The model under review builds one solid part; all positions refer to its coordinate system, in mm. Face numbers are marked on the shaded views. Round coordinates to 2 decimals unless told otherwise and drop trailing zeros. Answer as a JSON object with one key per item and string values. Group by question number.
Item 1: The part is to be moulded in two halves that separate along Y. For the marked faces 1, 2, 3 and 4, say which applies: +Y half, -Y half, draft (parallel to the pull), parting line (faces both ways), or undercut.
Item 2: To check wall thickness, follow line 1 (Y direction, x = -14.5, z = 0); line 2 (Z direction, x = -11, y = -6); line 3 (Z direction, x = -10.5, y = 11.5). State the ranges of each line that lie inside material, in increasing order.
Item 3: Insertion check: P1, Ø3, axis at x = -10.5, y = 1, coming from the -Z side; P2, Ø3, axis at y = 13.5, z = 0, coming from the +X side; P3, Ø4, axis at x = -5, y = 6.5, coming from the -Z side; P4, Ø5.5, axis at y = 3, z = 1.5, coming from the +X side. Each pin has a flat end and moves straight along its axis. Give the tip position at first contact, or say it passes through.
Item 4: Consider section A-A (y = 1). State how many separate pieces and enclosed holes the cut face has, and give its area (3 significant figures).
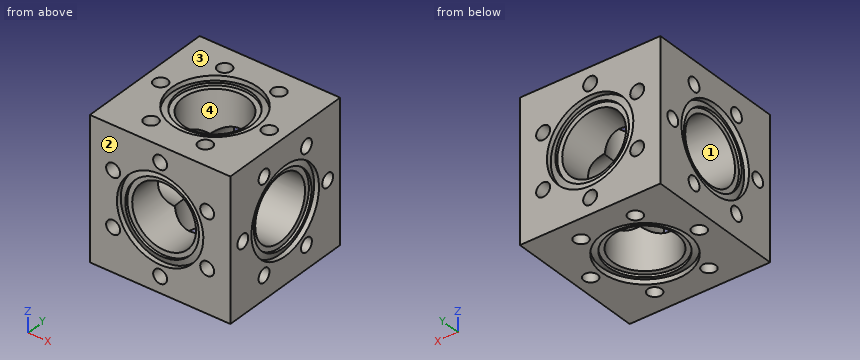
```python
from build123d import *

# Parameters (mm, degrees)
SKETCH1_W           = 34.925
SKETCH1_H           = 34.925
BOSS_EXTRUDE1_DEPTH = 17.4625
CIRPATTERN1_COUNT   = 6
CIRPATTERN2_COUNT   = 6
CIRPATTERN3_COUNT   = 6
CIRPATTERN4_COUNT   = 4
CIRPATTERN5_COUNT   = 4


with BuildPart() as part:
    # Sketch1 → Boss-Extrude1 (new, symmetric)
    with BuildSketch(Plane.XY):
        Rectangle(SKETCH1_W, SKETCH1_H)
    extrude(amount=BOSS_EXTRUDE1_DEPTH, both=True)

    # Sketch6 → Cut-Revolve1 (revolve, cut)
    with BuildSketch(Plane.XY, mode=Mode.PRIVATE) as cut_revolve1_sk:
        Polygon((17.4625, 10.7442), (16.249697253, 10.7442), (16.8275, 9.1567), (16.1925, 9.1567), (16.1925, 7.9375), (0, 7.9375), (0, 0), (17.4625, 0), align=None)
    cut_revolve1 = revolve(cut_revolve1_sk.sketch.rotate(Axis((17.4625, 0, 0), (1, 0, 0)), 90), axis=Axis((17.4625, 0, 0), (1, 0, 0)), mode=Mode.SUBTRACT)

    # Sketch5 → Tapped Hole0 (revolve, cut)
    with BuildSketch(Plane(origin=(17.4625, 13.5001, 0), x_dir=(0, 0, -1), z_dir=(0, 1, 0))):
        Polygon((0, 0), (0, 7.387806428), (1.727199945, 6.35), (1.727199945, 0), align=None)
    tapped_hole0 = revolve(axis=Axis((23.8125, 13.5001, 0), (-1, 0, 0)), mode=Mode.SUBTRACT)

    # Sketch8 → Tapped Hole1 (revolve, cut)
    with BuildSketch(Plane(origin=(0, 17.4625, -13.5001), x_dir=(0, 0, 1), z_dir=(1, 0, 0))):
        Polygon((0, 0), (0, 7.387806428), (1.727199945, 6.35), (1.727199945, 0), align=None)
    tapped_hole1 = revolve(axis=Axis((0, 23.8125, -13.5001), (0, -1, 0)), mode=Mode.SUBTRACT)

    # Sketch10 → Tapped Hole2 (revolve, cut)
    with BuildSketch(Plane(origin=(13.5001, 0, 17.4625), x_dir=(0, -1, 0), z_dir=(1, 0, 0))):
        Polygon((0, 0), (0, 7.387806428), (1.727199945, 6.35), (1.727199945, 0), align=None)
    tapped_hole2 = revolve(axis=Axis((13.5001, 0, 23.8125), (0, 0, -1)), mode=Mode.SUBTRACT)

    # CirPattern1: Tapped Hole0 ×6 about axis
    cirpattern1_axis = Axis((0, 0, 0), (1, 0, 0))
    for i in range(1, CIRPATTERN1_COUNT):
        add(tapped_hole0.rotate(cirpattern1_axis, i * 360 / CIRPATTERN1_COUNT), mode=Mode.SUBTRACT)

    # CirPattern2: Tapped Hole1 ×6 about axis
    cirpattern2_axis = Axis((0, 0, 0), (0, 1, 0))
    for i in range(1, CIRPATTERN2_COUNT):
        add(tapped_hole1.rotate(cirpattern2_axis, i * 360 / CIRPATTERN2_COUNT), mode=Mode.SUBTRACT)

    # CirPattern3: Tapped Hole2 ×6 about axis
    cirpattern3_axis = Axis((0, 0, 0), (0, 0, 1))
    for i in range(1, CIRPATTERN3_COUNT):
        add(tapped_hole2.rotate(cirpattern3_axis, i * 360 / CIRPATTERN3_COUNT), mode=Mode.SUBTRACT)

    # CirPattern4: Cut-Revolve1 ×4 about axis
    cirpattern4_axis = Axis((0, 0, 0), (0, 1, 0))
    for i in range(1, CIRPATTERN4_COUNT):
        add(cut_revolve1.rotate(cirpattern4_axis, i * 360 / CIRPATTERN4_COUNT), mode=Mode.SUBTRACT)

    # CirPattern5: Cut-Revolve1 ×4 about axis, 1 skipped
    cirpattern5_axis = Axis((0, 0, 0), (0, 0, -1))
    add([cut_revolve1.rotate(cirpattern5_axis, i * 360 / CIRPATTERN5_COUNT) for i in range(1, CIRPATTERN5_COUNT) if i not in (2,)], mode=Mode.SUBTRACT)

    # Mirror1: Tapped Hole2 across plane
    add(tapped_hole2.mirror(Plane.XY), mode=Mode.SUBTRACT)

    # Mirror1 copy 1 sketch → Mirror1 copy 1 (revolve, cut)
    with BuildSketch(Plane(origin=(6.75005, 11.691429554, -17.4625), x_dir=(0.8660254037844386, -0.5000000000000001, 0), z_dir=(0.5000000000000001, 0.8660254037844386, 0))):
        Polygon((0, 0), (0, -7.387806428), (1.727199945, -6.35), (1.727199945, 0), align=None)
    revolve(axis=Axis((6.75005, 11.691429554, -23.8125), (0, 0, -1)), mode=Mode.SUBTRACT)

    # Mirror1 copy 2 sketch → Mirror1 copy 2 (revolve, cut)
    with BuildSketch(Plane(origin=(-6.75005, 11.691429554, -17.4625), x_dir=(0.8660254037844387, 0.4999999999999998, 0), z_dir=(-0.4999999999999998, 0.8660254037844387, 0))):
        Polygon((0, 0), (0, -7.387806428), (1.727199945, -6.35), (1.727199945, 0), align=None)
    revolve(axis=Axis((-6.75005, 11.691429554, -23.8125), (0, 0, -1)), mode=Mode.SUBTRACT)

    # Mirror1 copy 3 sketch → Mirror1 copy 3 (revolve, cut)
    with BuildSketch(Plane(origin=(-13.5001, 0, -17.4625), x_dir=(0, 1, 0), z_dir=(-1, 0, 0))):
        Polygon((0, 0), (0, -7.387806428), (1.727199945, -6.35), (1.727199945, 0), align=None)
    revolve(axis=Axis((-13.5001, 0, -23.8125), (0, 0, -1)), mode=Mode.SUBTRACT)

    # Mirror1 copy 4 sketch → Mirror1 copy 4 (revolve, cut)
    with BuildSketch(Plane(origin=(-6.75005, -11.691429554, -17.4625), x_dir=(-0.8660254037844384, 0.5000000000000004, 0), z_dir=(-0.5000000000000004, -0.8660254037844384, 0))):
        Polygon((0, 0), (0, -7.387806428), (1.727199945, -6.35), (1.727199945, 0), align=None)
    revolve(axis=Axis((-6.75005, -11.691429554, -23.8125), (0, 0, -1)), mode=Mode.SUBTRACT)

    # Mirror1 copy 5 sketch → Mirror1 copy 5 (revolve, cut)
    with BuildSketch(Plane(origin=(6.75005, -11.691429554, -17.4625), x_dir=(-0.8660254037844386, -0.5000000000000001, 0), z_dir=(0.5000000000000001, -0.8660254037844386, 0))):
        Polygon((0, 0), (0, -7.387806428), (1.727199945, -6.35), (1.727199945, 0), align=None)
    revolve(axis=Axis((6.75005, -11.691429554, -23.8125), (0, 0, -1)), mode=Mode.SUBTRACT)

    # Mirror2: Tapped Hole1 across plane
    add(tapped_hole1.mirror(Plane.ZX), mode=Mode.SUBTRACT)

    # Mirror2 copy 1 sketch → Mirror2 copy 1 (revolve, cut)
    with BuildSketch(Plane(origin=(-11.691429554, -17.4625, -6.75005), x_dir=(0.8660254037844386, 0, 0.5000000000000001), z_dir=(0.5000000000000001, 0, -0.8660254037844386))):
        Polygon((0, 0), (0, -7.387806428), (1.727199945, -6.35), (1.727199945, 0), align=None)
    revolve(axis=Axis((-11.691429554, -23.8125, -6.75005), (0, -1, 0)), mode=Mode.SUBTRACT)

    # Mirror2 copy 2 sketch → Mirror2 copy 2 (revolve, cut)
    with BuildSketch(Plane(origin=(-11.691429554, -17.4625, 6.75005), x_dir=(0.8660254037844387, 0, -0.4999999999999998), z_dir=(-0.4999999999999998, 0, -0.8660254037844387))):
        Polygon((0, 0), (0, -7.387806428), (1.727199945, -6.35), (1.727199945, 0), align=None)
    revolve(axis=Axis((-11.691429554, -23.8125, 6.75005), (0, -1, 0)), mode=Mode.SUBTRACT)

    # Mirror2 copy 3 sketch → Mirror2 copy 3 (revolve, cut)
    with BuildSketch(Plane(origin=(0, -17.4625, 13.5001), x_dir=(0, 0, -1), z_dir=(-1, 0, 0))):
        Polygon((0, 0), (0, -7.387806428), (1.727199945, -6.35), (1.727199945, 0), align=None)
    revolve(axis=Axis((0, -23.8125, 13.5001), (0, -1, 0)), mode=Mode.SUBTRACT)

    # Mirror2 copy 4 sketch → Mirror2 copy 4 (revolve, cut)
    with BuildSketch(Plane(origin=(11.691429554, -17.4625, 6.75005), x_dir=(-0.8660254037844384, 0, -0.5000000000000004), z_dir=(-0.5000000000000004, 0, 0.8660254037844384))):
        Polygon((0, 0), (0, -7.387806428), (1.727199945, -6.35), (1.727199945, 0), align=None)
    revolve(axis=Axis((11.691429554, -23.8125, 6.75005), (0, -1, 0)), mode=Mode.SUBTRACT)

    # Mirror2 copy 5 sketch → Mirror2 copy 5 (revolve, cut)
    with BuildSketch(Plane(origin=(11.691429554, -17.4625, -6.75005), x_dir=(-0.8660254037844386, 0, 0.5000000000000001), z_dir=(0.5000000000000001, 0, 0.8660254037844386))):
        Polygon((0, 0), (0, -7.387806428), (1.727199945, -6.35), (1.727199945, 0), align=None)
    revolve(axis=Axis((11.691429554, -23.8125, -6.75005), (0, -1, 0)), mode=Mode.SUBTRACT)

    # Mirror3: Tapped Hole0 across plane
    add(tapped_hole0.mirror(Plane(origin=(0, 0, 0), x_dir=(0, 0, 1), z_dir=(1, 0, 0))), mode=Mode.SUBTRACT)

    # Mirror3 copy 1 sketch → Mirror3 copy 1 (revolve, cut)
    with BuildSketch(Plane(origin=(-17.4625, 6.75005, 11.691429554), x_dir=(0, 0.8660254037844386, -0.5000000000000001), z_dir=(0, 0.5000000000000001, 0.8660254037844386))):
        Polygon((0, 0), (0, -7.387806428), (1.727199945, -6.35), (1.727199945, 0), align=None)
    revolve(axis=Axis((-23.8125, 6.75005, 11.691429554), (-1, 0, 0)), mode=Mode.SUBTRACT)

    # Mirror3 copy 2 sketch → Mirror3 copy 2 (revolve, cut)
    with BuildSketch(Plane(origin=(-17.4625, -6.75005, 11.691429554), x_dir=(0, 0.8660254037844387, 0.4999999999999998), z_dir=(0, -0.4999999999999998, 0.8660254037844387))):
        Polygon((0, 0), (0, -7.387806428), (1.727199945, -6.35), (1.727199945, 0), align=None)
    revolve(axis=Axis((-23.8125, -6.75005, 11.691429554), (-1, 0, 0)), mode=Mode.SUBTRACT)

    # Mirror3 copy 3 sketch → Mirror3 copy 3 (revolve, cut)
    with BuildSketch(Plane(origin=(-17.4625, -13.5001, 0), x_dir=(0, 0, 1), z_dir=(0, -1, 0))):
        Polygon((0, 0), (0, -7.387806428), (1.727199945, -6.35), (1.727199945, 0), align=None)
    revolve(axis=Axis((-23.8125, -13.5001, 0), (-1, 0, 0)), mode=Mode.SUBTRACT)

    # Mirror3 copy 4 sketch → Mirror3 copy 4 (revolve, cut)
    with BuildSketch(Plane(origin=(-17.4625, -6.75005, -11.691429554), x_dir=(0, -0.8660254037844384, 0.5000000000000004), z_dir=(0, -0.5000000000000004, -0.8660254037844384))):
        Polygon((0, 0), (0, -7.387806428), (1.727199945, -6.35), (1.727199945, 0), align=None)
    revolve(axis=Axis((-23.8125, -6.75005, -11.691429554), (-1, 0, 0)), mode=Mode.SUBTRACT)

    # Mirror3 copy 5 sketch → Mirror3 copy 5 (revolve, cut)
    with BuildSketch(Plane(origin=(-17.4625, 6.75005, -11.691429554), x_dir=(0, -0.8660254037844386, -0.5000000000000001), z_dir=(0, 0.5000000000000001, -0.8660254037844386))):
        Polygon((0, 0), (0, -7.387806428), (1.727199945, -6.35), (1.727199945, 0), align=None)
    revolve(axis=Axis((-23.8125, 6.75005, -11.691429554), (-1, 0, 0)), mode=Mode.SUBTRACT)


solid = part.part
```
Geometry results:
{
 "1": {"face 1": "undercut", "face 2": "-Y half", "face 3": "draft", "face 4": "undercut"},
 "2": {"line 1": "y = -17.46 to -15.23, -11.77 to -7.94, 7.94 to 11.77, 15.23 to 17.46", "line 2": "z = -17.46 to -13.04, -10.35 to -5.2, 5.2 to 10.35, 13.04 to 17.46", "line 3": "z = -17.46 to -8, -5.5 to 5.5, 8 to 17.46"},
 "3": {"P1": "stops at z = -17.46", "P2": "stops at x = 10.98", "P3": "stops at z = -16.83", "P4": "passes through"},
 "4": {"separate pieces": "4", "enclosed holes": "0", "area": "269 mm^2"}
}
